```python
from build123d import *

# Parameters (mm, degrees)
SKETCH_1_W      = 124
SKETCH_1_H      = 124
SKETCH_1_R      = 1.5
SKETCH_1_W_2    = 88
SKETCH_1_H_2    = 88
SKETCH_1_W_3    = 73.332050418
SKETCH_1_H_3    = 2.87064966
EXTRUDE_1_DEPTH = 0.5


with BuildPart() as part:
    # Эскиз1 → Бобышка-Вытянуть1 (new body)
    with BuildSketch(Plane(origin=(0, 0, 0), x_dir=(1, 0, 0), z_dir=(0, 1, 0))):
        with Locations((62, 62)):
            Rectangle(SKETCH_1_W, SKETCH_1_H)
        with Locations((4, 120)):
            Circle(SKETCH_1_R, mode=Mode.SUBTRACT)
        with Locations((120, 120)):
            Circle(SKETCH_1_R, mode=Mode.SUBTRACT)
        with Locations((120, 4)):
            Circle(SKETCH_1_R, mode=Mode.SUBTRACT)
        with Locations((4, 4)):
            Circle(SKETCH_1_R, mode=Mode.SUBTRACT)
        with Locations((62, 62)):
            Rectangle(SKETCH_1_W_2, SKETCH_1_H_2, mode=Mode.SUBTRACT)
        with Locations((56.855908172, 111.032001236)):
            Rectangle(SKETCH_1_W_3, SKETCH_1_H_3, mode=Mode.SUBTRACT)
    extrude(amount=EXTRUDE_1_DEPTH)


solid = part.part
```
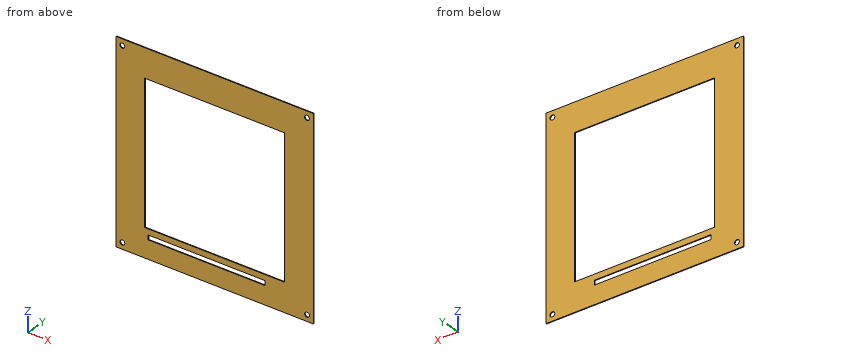
For this review, take the finished solid that the model builds, in its own axes (mm). Give positions to 0.01 mm unless a question says otherwise; leave off trailing zeros. Order: outer loops, then holes, each group sorted by start corner. A loop starts at its lowest first (then second) coordinate and runs counter-clockwise, first axis right, second up.
1) Take a section at D-D (y = 0.4). Give the boundary of the cut face in (x, z).
2) Wall thickness on line 1 (Z direction, x = 120, y = 0.25); line 2 (X direction, y = 0.25, z = -4); line 3 (Z direction, x = 28.5, y = 0.35): over which ranges is each line inside the solid? List them lowest first.
3) Take a section at B-B (x = 120). Give the boundary of the cut face in (y, z), then the cut area to 3 significant figures.
4) Take a section at C-C (z = -4). Give the boundary of the cut face in (x, y).
5) Insertion check: pin 1 (2.5 mm diameter, centred on x = 120, z = -4, fed in from -Y). The pin has a flat end and moves straight along its axis. Give the tip position at first contact, or say it passes through.
6) Take a section at A-A (z = -39). Give the boundary of the cut face in (x, y), then the cut area to 3 significant figures.
Derived:
1. outline: (0, -124) - (124, -124) - (124, 0) - (0, 0) - close; hole circle Ø3 at (4, -120); hole circle Ø3 at (4, -4); hole (18, -106) - (106, -106) - (106, -18) - (18, -18) - close; hole (20.19, -112.47) - (93.52, -112.47) - (93.52, -109.6) - (20.19, -109.6) - close; hole circle Ø3 at (120, -120); hole circle Ø3 at (120, -4)
2. line 1: z = -124 to -121.5, -118.5 to -5.5, -2.5 to 0
2. line 2: x = 0 to 2.5, 5.5 to 118.5, 121.5 to 124
2. line 3: z = -124 to -112.47, -109.6 to -106, -18 to 0
3. outline: (0, -124) - (0.5, -124) - (0.5, -121.5) - (0, -121.5) - close; (0, -118.5) - (0.5, -118.5) - (0.5, -5.5) - (0, -5.5) - close; (0, -2.5) - (0.5, -2.5) - (0.5, 0) - (0, 0) - close
3. area: 59.0 mm2
4. outline: (0, 0) - (2.5, 0) - (2.5, 0.5) - (0, 0.5) - close; (5.5, 0) - (118.5, 0) - (118.5, 0.5) - (5.5, 0.5) - close; (121.5, 0) - (124, 0) - (124, 0.5) - (121.5, 0.5) - close
5. pin 1: passes through
6. outline: (0, 0) - (18, 0) - (18, 0.5) - (0, 0.5) - close; (106, 0) - (124, 0) - (124, 0.5) - (106, 0.5) - close
6. area: 18.0 mm2
